Drawing for the job (mm, zero at the part's lowest x, y, z). A direction names the side the tool comes from. Give positions to 0.01 mm unless a question says otherwise; leave off trailing zeros. Write each loop counter-clockwise with the first axis right and the second up, starting at its lowest first coordinate (ties: lowest second). Pieces come first, ordered by that corner, then holes. Notation, with made-up numbers: M -15,82 L 24,82 A13 ccw 24,107 Z; hole C 18.25,2.5 d5. An arc over 180 degrees is marked long. Use a Markdown table: item, result. Add a question column.
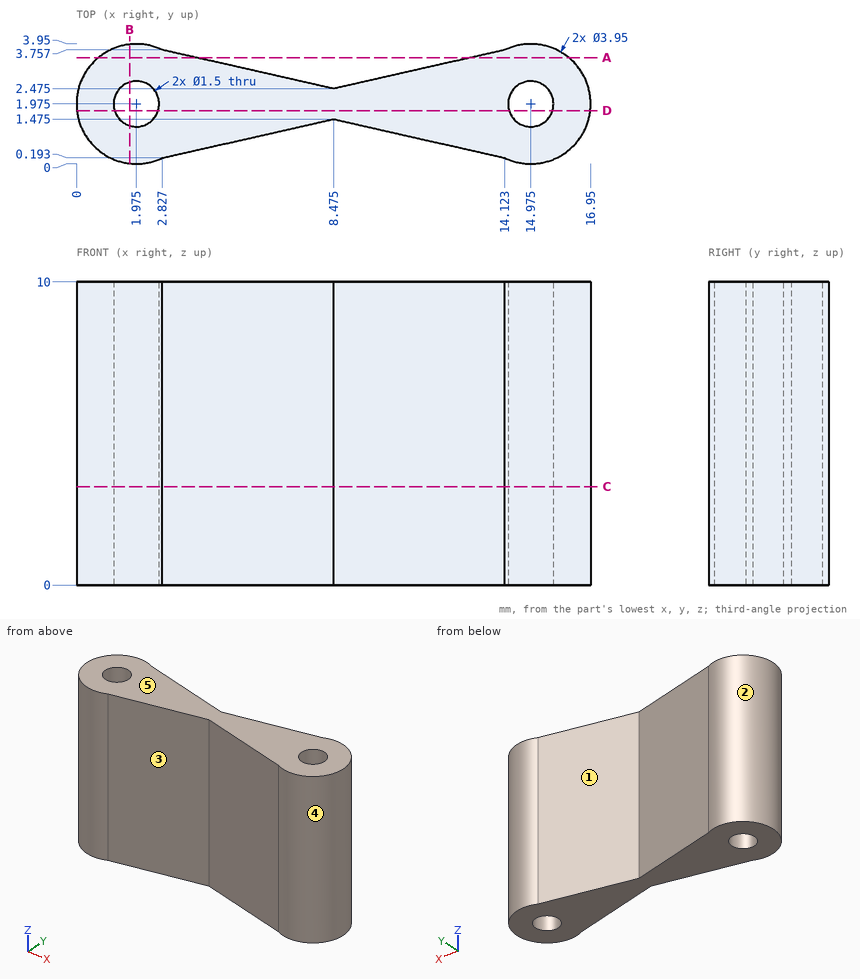
1. Cut at C-C (z = 3.25). Give the number of separate pieces and of enclosed holes in the cut face.
2. Cut at A-A (y = 3.5). Write the cut outline in (x, z).
3. Cut at B-B (x = 1.75). Write the cut outline in (y, z).
4. Drill centre lines: probe 1 along X at (y, z) = (1.75, 5.75); probe 2 along Y at (x, z) = (1.5, 8.5) (1 decimal); probe 3 along Y at (x, z) = (15.5, 4.75). Where is each one in solid material? Low to high. Write a range as [from, to].
5. Cut at D-D (y = 1.75). Write the cut outline in (x, z).
6. Mould opens along X. For the marked faces 4 and 5 say: released by +X, released by -X, zero draft, split by the parting line, or undercut.
7. Tool access for the marked faces 1, 2 and 3: list every direction of +Z, -Z, +X, -X, +Y, -Y with a clear straight run to the whole face (end or side of a thin tool).
8. Flat gauge pins, fed straight in: pin 1 (2 mm diameter, centred on x = 2, y = 2.5, fed in from -Z); pin 2 (1.5 mm diameter, centred on y = 3.5, z = 3.5, fed in from -X). Where does each tip first touch, or does it go through?
A:
| question | item | result |
|---|---|---|
| 1 | separate pieces | 1 |
| 1 | enclosed holes | 2 |
| 2 | outline | M 0.72,0 L 3.96,0 L 3.96,10 L 0.72,10 Z; M 12.99,0 L 16.23,0 L 16.23,10 L 12.99,10 Z |
| 3 | outline | M 0.01,0 L 1.26,0 L 1.26,10 L 0.01,10 Z; M 2.69,0 L 3.94,0 L 3.94,10 L 2.69,10 Z |
| 4 | probe 1 | x = [0.01, 1.26], [2.69, 14.26], [15.69, 16.94] |
| 4 | probe 2 | y = [0.1, 1.4], [2.6, 3.9] |
| 4 | probe 3 | y = [0.07, 1.44], [2.51, 3.88] |
| 5 | outline | M 0.01,0 L 1.26,0 L 1.26,10 L 0.01,10 Z; M 2.69,0 L 14.26,0 L 14.26,10 L 2.69,10 Z; M 15.69,0 L 16.94,0 L 16.94,10 L 15.69,10 Z |
| 6 | face 4 | undercut |
| 6 | face 5 | zero draft |
| 7 | face 1 | +Z, -Z, +Y |
| 7 | face 2 | +Z, -Z |
| 7 | face 3 | +Z, -Z, -Y |
| 8 | pin 1 | stops at z = 0 |
| 8 | pin 2 | stops at x = 0.16 |
